```python
from build123d import *

# Parameters (mm, degrees)
F1_DEPTH = 22.5
F2_DEPTH = 10
F0_W     = 12
F0_H     = 2.5
F3_DEPTH = 12.5
F4_DEPTH = 12.5
F5_DEPTH = 12.5


# Not quite as in the source:
# - a feature names something its author has since deleted; it is built from what else it names


with BuildPart() as f1:
    # F0 (on Front) → F1 (new body, symmetric)
    with BuildSketch(Plane.XZ):
        Polygon((8, 38.5), (8, 41), (-8, 41), (-8, 8), (-8, -27.5), (-8, -30), (-8, -38.5), (-5, -38.5), (-5, 38.5), (5, 38.5), (5, 34.5), align=None)
    extrude(amount=F1_DEPTH, both=True)

    # F0 (on Front) → F2 (join, symmetric)
    with BuildSketch(Plane.XZ):
        Polygon((-5, -38.5), (-8, -38.5), (-8, -41), (8, -41), (8, -38.5), (5, -34.5), (5, -38.5), align=None)
    extrude(amount=F2_DEPTH, both=True)

    # F0 (on Front) → F3 (join, symmetric)
    with BuildSketch(Plane.XZ):
        with Locations((-14, -28.75)):
            Rectangle(F0_W, F0_H)
    extrude(amount=F3_DEPTH, both=True)

    # F0 (on Front) → F4 (join, symmetric)
    with BuildSketch(Plane.XZ):
        Polygon((-20, -30), (-20, -27.5), (-20, 5), (-70, 5), (-70, -30), (-44.4338369071, -30), align=None)
        Polygon((-21, 4), (-21, -27.5), (-21, -29), (-45, -29), (-69, -29), (-69, 4), align=None, mode=Mode.SUBTRACT)
    extrude(amount=F4_DEPTH, both=True)

    # F0 (on Front) → F5 (join, symmetric)
    with BuildSketch(Plane.XZ):
        Polygon((-21, -29), (-21, -27.5), (-44.5986762643, -27.5), (-45, -29), align=None)
    extrude(amount=F5_DEPTH, both=True)


solid = f1.part
```
For this review, take the finished solid that the model builds, in its own axes (mm). A direction names the side the tool comes from. Give positions to 0.01 mm unless a question says otherwise; leave off trailing zeros. Order: outer loops, then holes, each group sorted by start corner. A loop starts at its lowest first (then second) coordinate and runs counter-clockwise, first axis right, second up.
1) Take a section at D-D (x = -61). Give the boundary of the cut face in (y, z).
2) Take a section at B-B (y = -9). Give the boundary of the cut face in (x, z).
3) Take a section at C-C (z = -10.5). Give the boundary of the cut face in (x, y).
4) Take a section at A-A (x = -41). Give the boundary of the cut face in (y, z).
5) For faces 1 (the face through (-45, 0, 5)), 2 (the face through (2, -10, -39)), 3 (the face through (-7, -16, -38.5)), 4 (the face through (5, 0, 37)), 5 (the face through (2, 10, -39)), list the 3-axis set-ups (+Z, -Z, +X, -X, +Y, -Y) from which the entire face can be reached by the end or side of a thin tool; tool diameter is ignored.
6) Wall thickness on line 1 (X direction, y = 4, z = 2.5); line 2 (Z direction, x = -30.5, y = -10); line 3 (Z direction, x = -47.5, y = 3): over which ranges is each line inside the solid? List them lowest first.
7) The part is to be moulded in two halves that separate along X. For faces 6 (the face through (-5.4, -22.5, 7.3)), 7 (the face through (-33, 0, -27.5)), 8 (the face through (6.5, -0.1, -36.5)), say which applies: released by +X, released by -X, zero draft, split by the parting line, or undercut.
8) Insertion check: pin 1 (1 mm diameter, centred on y = 9.5, z = 8, fed in from -X); pin 2 (6 mm diameter, centred on x = -16.5, y = -4, fed in from +Z); pin 3 (1 mm diameter, centred on x = -52.5, y = 7, fed in from +Z). Each pin has a flat end and moves straight along its axis. Give the tip position at first contact, or say it passes through.
Derived:
1. outline: (-12.5, -30) - (12.5, -30) - (12.5, -29) - (-12.5, -29) - close; (-12.5, 4) - (12.5, 4) - (12.5, 5) - (-12.5, 5) - close
2. outline: (-70, -30) - (-8, -30) - (-8, -41) - (8, -41) - (8, -38.5) - (5, -34.5) - (5, -38.5) - (-5, -38.5) - (-5, 38.5) - (5, 38.5) - (5, 34.5) - (8, 38.5) - (8, 41) - (-8, 41) - (-8, -27.5) - (-20, -27.5) - (-20, 5) - (-70, 5) - close; hole (-69, -29) - (-45, -29) - (-44.6, -27.5) - (-21, -27.5) - (-21, 4) - (-69, 4) - close
3. outline: (-70, -12.5) - (-69, -12.5) - (-69, 12.5) - (-70, 12.5) - close; (-21, -12.5) - (-20, -12.5) - (-20, 12.5) - (-21, 12.5) - close; (-8, -22.5) - (-5, -22.5) - (-5, 22.5) - (-8, 22.5) - close
4. outline: (-12.5, -30) - (12.5, -30) - (12.5, -27.5) - (-12.5, -27.5) - close; (-12.5, 4) - (12.5, 4) - (12.5, 5) - (-12.5, 5) - close
5. face 1: +Z, -X, +Y, -Y
5. face 2: -Z, +X, -Y
5. face 3: -Z, +X, -X, -Y
5. face 4: +Y, -Y
5. face 5: -Z, +X, +Y
6. line 1: x = -70 to -69, -21 to -20, -8 to -5
6. line 2: z = -30 to -27.5, 4 to 5
6. line 3: z = -30 to -29, 4 to 5
7. face 6: zero draft
7. face 7: undercut
7. face 8: released by +X
8. pin 1: stops at x = -8
8. pin 2: stops at z = -27.5
8. pin 3: stops at z = 5
